For this review, take the finished solid that the model builds, in its own axes (mm). Face numbers are marked on the shaded views. Coordinates: 2 decimals unless noted, no trailing zeros. Order: outer loops, then holes, each group sorted by start corner. A loop starts at its lowest first (then second) coordinate and runs counter-clockwise, first axis right, second up. Notation, with made-up numbers: (13.25, 12) - (23.25, 12) arc R31 cw to (23.25, 39) - close; hole circle Ø1 at (-2, -6). An arc over 180 degrees is marked (long way). One line per item, written item: value. Start each with the question number.
(1) Consider section C-C on x = 0. Write out the cut boundary in (y, z), then the cut area to 3 significant figures.
(2) Mouldability with a two-part tool opening along Z and no side actions: class the marked faces 1, 2, 3 and 4 as released by +Z, released by -Z, zero draft, split by the parting line, or undercut.
(3) Consider section D-D on z = 0. Write out the cut boundary in (x, y).
(4) Consider section B-B on x = 25. Write out the cut boundary in (y, z).
(5) Consider section A-A on z = 25. Write out the cut boundary in (x, y), then the cut area to 3 significant figures.
(6) To check wall thickness, follow line 1 along Z through (x, y) = (-0.5, 12.5); line 2 along X through (y, z) = (4.5, -25); line 3 along X through (y, z) = (2.5, 4.5). State the ranges of each line that lie inside material, in increasing order.
(7) Clearance check with a flat-ended pin moving along its axis: pin 1 (7 mm diameter, centred on x = 1.5, z = 3, fed in from -Y). State where the tip first meets the part, or that it passes through.
```python
from build123d import *

# Parameters (mm, degrees)
SKETCH1_R           = 7
SKETCH1_R_2         = 2
BOSS_EXTRUDE1_DEPTH = 15
BOSS_EXTRUDE2_START = -8
SKETCH2_R           = 7
SKETCH2_R_2         = 5.5
BOSS_EXTRUDE2_DEPTH = 8


with BuildPart() as part:
    # Sketch1 → Boss-Extrude1 (new body)
    with BuildSketch(Plane(origin=(0, 0, 0), x_dir=(1, 0, 0), z_dir=(0, 1, 0))):
        with BuildLine():
            Line((-30, 40), (30, 40))
            ThreePointArc((30, 40), (37.071067812, 37.071067812), (40, 30))
            Line((40, 30), (40, -30))
            ThreePointArc((40, -30), (37.071067812, -37.071067812), (30, -40))
            Line((30, -40), (-30, -40))
            ThreePointArc((-30, -40), (-37.071067812, -37.071067812), (-40, -30))
            Line((-40, -30), (-40, 30))
            ThreePointArc((-40, 30), (-37.071067812, 37.071067812), (-30, 40))
        make_face()
        with Locations(Location((0, 0, 0), (0, 0, 270))):
            Circle(SKETCH1_R, mode=Mode.SUBTRACT)
        with Locations(Location((0, 25, 0), (0, 0, 270))):
            Circle(SKETCH1_R_2, mode=Mode.SUBTRACT)
        with Locations(Location((0, -25, 0), (0, 0, 270))):
            Circle(SKETCH1_R_2, mode=Mode.SUBTRACT)
        with Locations(Location((-25, 0, 0), (0, 0, 270))):
            Circle(SKETCH1_R_2, mode=Mode.SUBTRACT)
        with Locations(Location((25, 0, 0), (0, 0, 270))):
            Circle(SKETCH1_R_2, mode=Mode.SUBTRACT)
    extrude(amount=BOSS_EXTRUDE1_DEPTH)

    # Sketch2 → Boss-Extrude2 (add)
    with BuildSketch(Plane(origin=(0, 15, 0), x_dir=(1, 0, 0), z_dir=(0, 1, 0)).offset(BOSS_EXTRUDE2_START)):
        with Locations(Location((0, 0, 0), (0, 0, 270))):
            Circle(SKETCH2_R)
        with Locations(Location((0, 0, 0), (0, 0, 270))):
            Circle(SKETCH2_R_2, mode=Mode.SUBTRACT)
    extrude(amount=BOSS_EXTRUDE2_DEPTH)


solid = part.part
```
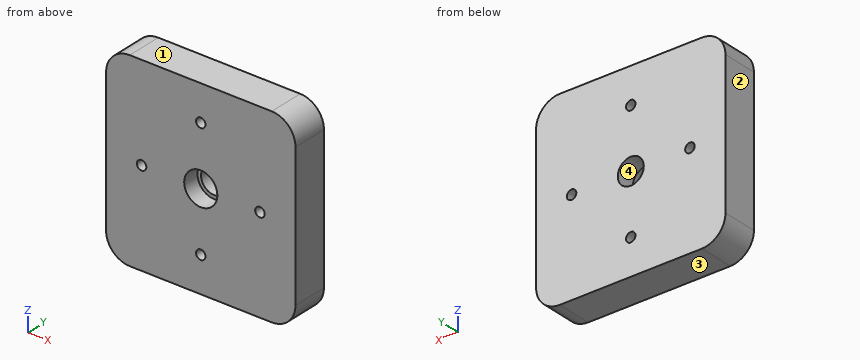
Geometry check:
1. outline: (0, -40) - (15, -40) - (15, -27) - (0, -27) - close; (0, -23) - (15, -23) - (15, -5.5) - (7, -5.5) - (7, -7) - (0, -7) - close; (0, 7) - (7, 7) - (7, 5.5) - (15, 5.5) - (15, 23) - (0, 23) - close; (0, 27) - (15, 27) - (15, 40) - (0, 40) - close
1. area: 894 mm^2
2. face 1: released by +Z
2. face 2: zero draft
2. face 3: released by -Z
2. face 4: undercut
3. outline: (-40, 0) - (-27, 0) - (-27, 15) - (-40, 15) - close; (-23, 0) - (-7, 0) - (-7, 7) - (-5.5, 7) - (-5.5, 15) - (-23, 15) - close; (5.5, 7) - (7, 7) - (7, 0) - (23, 0) - (23, 15) - (5.5, 15) - close; (27, 0) - (40, 0) - (40, 15) - (27, 15) - close
4. outline: (0, -40) - (15, -40) - (15, -2) - (0, -2) - close; (0, 2) - (15, 2) - (15, 40) - (0, 40) - close
5. outline: (-40, 0) - (-2, 0) - (-2, 15) - (-40, 15) - close; (2, 0) - (40, 0) - (40, 15) - (2, 15) - close
5. area: 1,140 mm^2
6. line 1: z = -40 to -26.94, -23.06 to -5.48, 5.48 to 23.06, 26.94 to 40
6. line 2: x = -40 to -2, 2 to 40
6. line 3: x = -40 to -5.36, 5.36 to 40
7. pin 1: stops at y = 7
